Autodesk Inventor part; units mm, degrees
ref_plane "YZ Plane" through (0, 0, 0) normal (1, 0, 0) x (0, 1, 0)
ref_plane "XY Plane" through (0, 0, 0) normal (0, 0, 1) x (1, 0, 0)
sketch "Sketch1" plane through (0, 0, 0) normal (0, 0, 1) x (1, 0, 0)
  line L0 (0, 0) -> (30, 0)
  line L1 (30, 0) -> (30, 30)
  line L2 (30, 30) -> (0, 30)
  line L3 (0, 30) -> (0, 0)
  dimension "d0" = 30
  dimension "d1" = 30
extrude "Extrusion1" add sketch "Sketch1" along normal mid plane 120
ref_plane "Work Plane1" through (0, 15, 0) normal (0, 1, 0) x (-1, 0, 0)
split body "Split1" result two bodies by plane through (0, 15, 0) normal (0, 1, 0) first body at (20, 15.5, -20)
combine bodies "Combine1" operation type add bodies to combine 3 2
shell "Shell1" thickness 1 removed faces 1 at (10, 30, 20) bodies 2
properties part number "excersise 3"
Geometry: final body of the model. Coordinates: model frame, mm. A direction names the side the tool comes from. Round coordinates to 2 decimals unless told otherwise and drop trailing zeros. Order: outer loops, then holes, each group sorted by start corner. A loop starts at its lowest first (then second) coordinate and runs counter-clockwise, first axis right, second up. Notation, with made-up numbers: (4.25, -24.5) -> (33.25, -24.5) arc R20 cw to (33.25, -2.5) -> close; hole circle Ø9 at (35, -16.5). An arc over 180 degrees is marked (long way). Put each result on its own line as item: value. Start each with the question number.
Q1. Pull-direction query (Z, two-part tool) for faces 1 (the flat face through (15, 16, 59)), 2 (the flat face through (15, 0, -1)), 3 (the flat face through (15, 15, -60)); classes: +Z half, -Z half, draft (parallel to the pull), parting line (faces both ways), or undercut.
Q2. Section C-C on y = 9.25. Return the cut outline in (x, z).
Q3. Section A-A on x = 11.25. Return the cut outline in (y, z).
Q4. Section B-B on z = -36.5. Return the cut outline in (x, y).
Q5. Reachability of faces 4 (the flat face through (1, 16, -1)), 5 (the flat face through (29.5, 30, -0.3)) from +Z, -Z, +X, -X, +Y, -Y: full face, straight path, thin tool, end or side. Return the list, or none.
Q6. Line query: probe 1 along Z at (x, y) = (8.75, 16); probe 2 along X at (y, z) = (17.75, -16.5); probe 3 along Y at (x, z) = (19.5, -48.5). Output: solid intervals per line, ascending.
Q7. First-contact query: pin 1 (6 mm diameter, centred on x = 7, z = 30, fed in from +Y); pin 2 (1.5 mm diameter, centred on x = 15, z = 41, fed in from -Y). Flat tips, straight axial feed; report the tip coordinate or a pass-through.
Ans:
1. face 1: undercut
1. face 2: draft
1. face 3: -Z half
2. outline: (0, -60) -> (30, -60) -> (30, 60) -> (0, 60) -> close; hole (1, -59) -> (29, -59) -> (29, 59) -> (1, 59) -> close
3. outline: (0, -60) -> (30, -60) -> (30, -59) -> (1, -59) -> (1, 59) -> (30, 59) -> (30, 60) -> (0, 60) -> close
4. outline: (0, 0) -> (30, 0) -> (30, 30) -> (29, 30) -> (29, 1) -> (1, 1) -> (1, 30) -> (0, 30) -> close
5. face 4: +Y
5. face 5: +Z, -Z, +X, -X, +Y
6. probe 1: z = -60 to -59, 59 to 60
6. probe 2: x = 0 to 1, 29 to 30
6. probe 3: y = 0 to 1
7. pin 1: stops at y = 1
7. pin 2: stops at y = 0
